Autodesk Inventor part; units mm, degrees
ref_plane "YZ Plane" through (0, 0, 0) normal (1, 0, 0) x (0, 1, 0)
ref_plane "XZ Plane" through (0, 0, 0) normal (0, 1, 0) x (-1, 0, 0)
ref_plane "XY Plane" through (0, 0, 0) normal (0, 0, 1) x (1, 0, 0)
sketch "Sketch1" plane through (0, 0, 0) normal (0, 1, 0) x (-1, 0, 0)
  line L0 (-26.9875, 42.8625) -> (26.9875, 42.8625)
  line L1 (26.9875, 42.8625) -> (26.9875, -42.8625)
  line L2 (26.9875, -42.8625) -> (-26.9875, -42.8625)
  line L3 (-26.9875, -42.8625) -> (-26.9875, 42.8625)
  line L4 (-26.9875, 42.8625) -> (26.9875, -42.8625) construction
  line L5 (26.9875, 42.8625) -> (-26.9875, -42.8625) construction
  point P0 (0, 0)
  dimension "d0" = 53.975
  dimension "d1" = 85.725
extrude "Extrusion1" add sketch "Sketch1" along normal blind 1.57
sketch "Sketch2" plane through (0, 1.57, 0) normal (0, 1, 0) x (1, 0, 0)
  line L0 (-26.9875, -42.8625) -> (26.9875, -42.8625)
  line L1 (-26.9875, 42.8625) -> (-26.9875, -42.8625)
  line L2 (26.9875, 42.8625) -> (-26.9875, 42.8625)
  line L3 (26.9875, -42.8625) -> (26.9875, 42.8625)
  point P0 (0, 0)
  point P1 (-22.9235, -38.7985)
  point P2 (-22.9235, 38.7985)
  dimension "d4" = 4.064
  dimension "d5" = 4.064
  dimension "d6" = 4.064
  dimension "d7" = 4.064
hole "Hole1" at (-22.9235, 1.57, 38.7985) at (-22.9235, 1.57, -38.7985) direction (0, -1, 0) diameter 3 depth 2.54
sketch "Sketch5" plane through (0, 1.57, 0) normal (0, 1, 0) x (1, 0, 0)
  line L0 (-26.9875, -42.8625) -> (26.9875, -42.8625)
  line L1 (26.9875, -42.8625) -> (26.9875, 42.8625)
  line L2 (-4.9284, -30.8693) -> (-9.1184, -30.8693)
  line L3 (-9.1184, -30.8693) -> (-9.1184, -36.0693)
  line L4 (-9.1184, -36.0693) -> (-4.9284, -36.0693)
  line L5 (-4.9284, -36.0693) -> (-4.9284, -30.8693)
  line L6 (-4.9284, -30.8693) -> (-9.1184, -36.0693) construction
  line L7 (-9.1184, -30.8693) -> (-4.9284, -36.0693) construction
  point P0 (0, 0)
  point P1 (-7.3025, -33.9725)
  point P2 (-7.0234, -33.4693)
  dimension "d26" = 8.89
  dimension "d27" = 34.29
  dimension "d28" = 5.2
  dimension "d29" = 4.19
extrude "Extrusion4" add sketch "Sketch5" along normal blind 8.77
sketch "Sketch6" plane through (0, 1.57, 0) normal (0, 1, 0) x (1, 0, 0)
  line L0 (-6.0004, 7.1846) -> (-24.0004, 7.1846)
  line L1 (-24.0004, 7.1846) -> (-24.0004, 32.6846)
  line L2 (-24.0004, 32.6846) -> (-6.0004, 32.6846)
  line L3 (-6.0004, 32.6846) -> (-6.0004, 7.1846)
  line L4 (-6.0004, 7.1846) -> (-24.0004, 32.6846) construction
  line L5 (-24.0004, 7.1846) -> (-6.0004, 32.6846) construction
  point P0 (0, 0)
  point P1 (-15.0004, 19.9346)
  dimension "d34" = 25.5
  dimension "d35" = 18
extrude "Extrusion5" add sketch "Sketch6" along normal blind 4.2
sketch "Sketch7" plane through (0, 0, 0) normal (0, -1, 0) x (1, 0, 0)
  line L0 (2.7595, 37.1835) -> (-3.1405, 37.1835)
  line L1 (-3.1405, 37.1835) -> (-3.1405, 41.6835)
  line L2 (-3.1405, 41.6835) -> (2.7595, 41.6835)
  line L3 (2.7595, 41.6835) -> (2.7595, 37.1835)
  line L4 (2.7595, 37.1835) -> (-3.1405, 41.6835) construction
  line L5 (-3.1405, 37.1835) -> (2.7595, 41.6835) construction
  line L6 (-26.9875, 42.8625) -> (26.9875, 42.8625)
  line L7 (-26.9875, -42.8625) -> (-26.9875, 42.8625)
  line L8 (26.9875, 42.8625) -> (26.9875, -42.8625)
  point P0 (0, 0)
  point P1 (-0.1905, 39.4335)
  dimension "d36" = 4.5
  dimension "d37" = 5.9
  dimension "d38" = 3.429
  dimension "d40" = 27.178
extrude "Extrusion6" add sketch "Sketch7" along normal blind 6
sketch "Sketch8" plane through (0, 1.57, 0) normal (0, 1, 0) x (1, 0, 0)
  line L0 (26.0985, -42.6085) -> (16.2941, -42.6085)
  line L1 (16.2941, -42.6085) -> (16.2941, -32.7279)
  line L2 (16.2941, -32.7279) -> (26.0985, -32.7279)
  line L3 (26.0985, -32.7279) -> (26.0985, -42.6085)
  line L4 (26.0985, -42.6085) -> (16.2941, -32.7279) construction
  line L5 (16.2941, -42.6085) -> (26.0985, -32.7279) construction
  line L6 (26.9875, -42.8625) -> (26.9875, 42.8625)
  line L7 (-26.9875, -42.8625) -> (26.9875, -42.8625)
  point P0 (0, 0)
  point P1 (21.1963, -37.6682)
  dimension "d43" = 9.8044
  dimension "d44" = 9.8806
  dimension "d45" = 0.889
  dimension "d46" = 0.254
extrude "Extrusion7" add sketch "Sketch8" along normal blind 6.1722
sketch "Sketch9" plane through (16.2941, 1.57, 42.6085) normal (0, 0, 1) x (1, 0, 0)
  line L0 (0, 0) -> (0, 6.1722)
  line L1 (7.0358, 4.2799) -> (2.2606, 4.2799)
  line L2 (2.2606, 4.2799) -> (2.2606, 1.8923)
  line L3 (2.2606, 1.8923) -> (7.0358, 1.8923)
  line L4 (7.0358, 1.8923) -> (7.0358, 4.2799)
  line L5 (7.0358, 4.2799) -> (2.2606, 1.8923) construction
  line L6 (2.2606, 4.2799) -> (7.0358, 1.8923) construction
  line L7 (0, 6.1722) -> (9.8044, 6.1722)
  point P0 (-16.2941, -1.57)
  point P1 (4.6482, 3.0861)
  dimension "d52" = 3.0861
  dimension "d53" = 2.2606
extrude "Extrusion8" add sketch "Sketch9" along normal blind 2.4892
sketch "Sketch10" plane through (0, 1.57, 0) normal (0, 1, 0) x (1, 0, 0)
  line L0 (26.9875, -42.8625) -> (26.9875, 42.8625)
  line L1 (-26.9875, -42.8625) -> (26.9875, -42.8625)
  line L2 (13.0175, -42.2275) -> (5.3975, -42.2275)
  line L3 (5.3975, -42.2275) -> (5.3975, -37.1475)
  line L4 (5.3975, -37.1475) -> (13.0175, -37.1475)
  line L5 (13.0175, -37.1475) -> (13.0175, -42.2275)
  line L6 (13.0175, -42.2275) -> (5.3975, -37.1475) construction
  line L7 (5.3975, -42.2275) -> (13.0175, -37.1475) construction
  point P0 (0, 0)
  point P1 (9.2075, -39.6875)
  dimension "d56" = 17.78
  dimension "d57" = 3.175
  dimension "d58" = 7.62
  dimension "d59" = 5.08
extrude "Extrusion9" add sketch "Sketch10" along normal blind 1.8
sketch "Sketch11" plane through (0, 1.57, 0) normal (0, 1, 0) x (1, 0, 0)
  line L0 (26.9875, -42.8625) -> (26.9875, 42.8625)
  line L1 (26.9875, 42.8625) -> (-26.9875, 42.8625)
  circle A0 centre (23.3172, 34.1249) radius 1.524
  circle A1 centre (-1.6764, 34.1249) radius 1.524
  point P0 (0, 0)
  dimension "d62" = 3.6703
  dimension "d63" = 24.9936
  dimension "d64" = 8.7376
  dimension "d65" = 8.7376
  dimension "d66" = 3.048
  dimension "d67" = 3.048
sketch "Sketch12" plane through (0, 1.57, 0) normal (0, 1, 0) x (1, 0, 0)
  line L0 (26.9875, -42.8625) -> (26.9875, 42.8625)
  line L1 (26.9875, 34.1249) -> (26.2255, 34.1249)
  line L2 (26.9875, 34.1249) -> (27.7495, 34.1249) construction
  line L3 (26.9875, 42.8625) -> (-26.9875, 42.8625)
  line L4 (26.2255, 34.1249) -> (26.2255, 31.1785)
  line L5 (26.2255, 31.1785) -> (-4.5847, 31.1785)
  line L6 (-4.5847, 31.1785) -> (-4.5847, 43.6245)
  line L7 (-4.5847, 43.6245) -> (26.2255, 43.6245)
  line L8 (26.2255, 43.6245) -> (26.2255, 31.1785)
  point P0 (0, 0)
  point P1 (26.2255, 42.8625)
  point P2 (-4.5847, 42.8625)
  dimension "d68" = 0.762
  dimension "d69" = 180
  dimension "d70" = 8.7376
  dimension "d73" = 2.9464
  dimension "d74" = 30.8102
  dimension "d75" = 12.446
extrude "Extrusion10" add sketch "Sketch12" along normal blind 12.5476 contours L4 L5 L6 L3 L8 | L3 L6 L7 L8
sketch "Sketch15" plane through (26.2255, 1.57, -43.6245) normal (0, 0, -1) x (-1, 0, 0)
  line L0 (23.5585, 2.3241) -> (7.2517, 2.3241)
  line L1 (7.2517, 2.3241) -> (7.2517, 10.2235)
  line L2 (7.2517, 10.2235) -> (23.5585, 10.2235)
  line L3 (23.5585, 10.2235) -> (23.5585, 2.3241)
  line L4 (23.5585, 2.3241) -> (7.2517, 10.2235) construction
  line L5 (7.2517, 2.3241) -> (23.5585, 10.2235) construction
  line L6 (30.8102, 0) -> (30.8102, 12.5476)
  line L7 (0, 12.5476) -> (30.8102, 12.5476)
  point P0 (26.2255, -1.57)
  point P1 (26.9875, 0)
  point P2 (15.4051, 6.2738)
  point P3 (30.8102, 6.2738)
  point P4 (15.4051, 12.5476)
  dimension "d86" = 16.3068
  dimension "d87" = 7.8994
extrude "Extrusion13" add sketch "Sketch15" along normal blind 6.0452
sketch "Sketch16" plane through (0, 14.1176, 0) normal (0, 1, 0) x (1, 0, 0)
  line L0 (26.2255, 43.6245) -> (-4.5847, 43.6245)
  line L1 (-1.9136, 43.6245) -> (-1.9136, 40.0431)
  line L2 (-1.9136, 43.6245) -> (1.6678, 43.6245) construction
  line L3 (22.654, 43.6245) -> (22.654, 40.0431)
  line L4 (26.2255, 42.8625) -> (26.2255, 31.1785)
  line L5 (18.9738, 43.6245) -> (18.9738, 49.6697)
  line L6 (26.2255, 31.1785) -> (-4.5847, 31.1785)
  line L7 (-4.5847, 43.6245) -> (-4.5847, 31.1785)
  line L8 (2.667, 43.6245) -> (2.667, 49.6697)
  line L9 (18.9738, 40.0431) -> (26.2255, 40.0431)
  line L10 (18.9738, 40.0431) -> (18.9738, 31.1785)
  line L11 (2.667, 40.0431) -> (-4.5847, 40.0431)
  line L12 (-4.5847, 31.1785) -> (-4.5847, 42.8625)
  line L13 (2.667, 40.0431) -> (2.667, 31.1785)
  point P0 (0, 0)
  dimension "d90" = 3.5814
  dimension "d91" = 270
  dimension "d92" = 3.5814
extrude "Extrusion14" cut sketch "Sketch16" against normal blind 8.9662 contours L9 L4 L6 L10 | L11 L13 L6 L7
extrude "Extrusion15" cut sketch "Sketch11" along normal mid plane 8.9662
properties part number "Spo2 PCB"
CAD build for the part. Positions are in the model's coordinates, mm. A direction names the side the tool comes from. Coordinates: 2 decimals unless noted, no trailing zeros. Write each loop counter-clockwise with the first axis right and the second up, starting at its lowest first coordinate (ties: lowest second). Pieces come first, ordered by that corner, then holes.
(1) Cut at B-B, the plane z = -18. List the corners of the cut face in (x, y), and give its area (3 significant figures).
(2) Cut at C-C, the plane z = -39. List the corners of the cut face in (x, y), and give its area (3 significant figures).
(3) Flat gauge pins, fed straight in: pin 1 (3.5 mm diameter, centred on y = 4, z = -24, fed in from +X); pin 2 (1.9 mm diameter, centred on y = 4.5, z = 40, fed in from +X); pin 3 (4.5 mm diameter, centred on y = 10.5, z = -35, fed in from -X); pin 4 (10 mm diameter, centred on y = 7, z = 6, fed in from +X). Where does each tip first touch, or does it go through?
(4) Cut at D-D, the plane x = 7. List the corners of the cut face in (y, z).
(5) Two-plate mould, pull along Z, no slides. Class faces 4 (the face through (-15, 4, -32.685)), 5 (the face through (-2.007, 2.612, -32.637)), 6 (the face through (11, 11.794, -47)): +Z half, -Z half, draft (parallel to the pull), parting line (faces both ways), or undercut.
(6) Drill centre lines: probe 1 along Y at (x, z) = (23, 37); probe 2 along Y at (x, z) = (17, -26); probe 3 along Z at (x, y) = (6, 13). Where is each one in solid material? Low to high.
(7) Cut at A-A, the plane x = -12. List the corners of the cut face in (y, z), and give its area (3 significant figures).
(8) 3-axis set-ups, long thin cutter, end or side, ignore diameter. For faces 1 (the face through (-1, 5.151, -36)), 2 (the face through (18.974, 10, -36)), 3 (the face through (-7, 6, 30.869)): which of +Z, -Z, +X, -X, +Y, -Y reach the whole face in a straight line?
Geometry says:
1. outline: (-26.99, 0) - (26.99, 0) - (26.99, 1.57) - (-6, 1.57) - (-6, 5.77) - (-24, 5.77) - (-24, 1.57) - (-26.99, 1.57) - close
1. area: 160 mm2
2. outline: (-26.99, 0) - (-24.41, 0) - (-24.41, 1.57) - (-26.99, 1.57) - close; (-21.44, 0) - (26.99, 0) - (26.99, 1.57) - (26.23, 1.57) - (26.23, 5.15) - (18.97, 5.15) - (18.97, 14.12) - (2.67, 14.12) - (2.67, 5.15) - (-4.58, 5.15) - (-4.58, 1.57) - (-21.44, 1.57) - close
2. area: 337 mm2
3. pin 1: stops at x = -6
3. pin 2: stops at x = 26.1
3. pin 3: stops at x = 2.67
3. pin 4: passes through
4. outline: (0, -42.86) - (1.57, -42.86) - (1.57, -43.62) - (3.89, -43.62) - (3.89, -49.67) - (11.79, -49.67) - (11.79, -43.62) - (14.12, -43.62) - (14.12, -31.18) - (1.57, -31.18) - (1.57, 37.15) - (3.37, 37.15) - (3.37, 42.23) - (1.57, 42.23) - (1.57, 42.86) - (0, 42.86) - close
5. face 4: -Z half
5. face 5: undercut
5. face 6: draft
6. probe 1: y = 0 to 7.74
6. probe 2: y = 0 to 1.57
6. probe 3: z = -43.62 to -31.18
7. outline: (0, -42.86) - (1.57, -42.86) - (1.57, -32.68) - (5.77, -32.68) - (5.77, -7.18) - (1.57, -7.18) - (1.57, 42.86) - (0, 42.86) - close
7. area: 242 mm2
8. face 1: +Z, +Y
8. face 2: +X, +Y
8. face 3: +X, -X, +Y
